The listing builds one solid part. Answer for the finished solid, in the listing's coordinates (mm). A direction names the side the tool comes from. Round coordinates to 2 decimals unless told otherwise and drop trailing zeros. Loops run counter-clockwise (first coordinate to the right, second up) from the corner with the lowest first, then second, coordinate; pieces in that order, holes last. Notation, with made-up numbers: M 7,-19 L 62,-19 A10 cw 62,-14 Z; hole C 53.5,84 d7. An arc over 180 degrees is marked long. Answer as a JSON object with one key per item and string values.
```python
from build123d import *

# Parameters (mm, degrees)
BOSS_EXTRUDE1_DEPTH     = 0.762
SKETCH3_R               = 1.651
SKETCH3_R_2             = 1.1557
BOSS_EXTRUDE2_DEPTH     = 3.175
BOSS_EXTRUDE3_DEPTH     = 0.762
CUT_EXTRUDE1_DEPTH      = 7.703386756
CUT_EXTRUDE1_DEPTH_BACK = 7.703386756
SKETCH5_R               = 1.1557


with BuildPart() as part:
    # Sketch2 → Boss-Extrude1 (new body)
    with BuildSketch(Plane(origin=(0, 0, 0), x_dir=(1, 0, 0), z_dir=(0, 1, 0))):
        with BuildLine():
            ThreePointArc((2.867741935, -1.88005784), (5.08, 0), (2.867741935, 1.88005784))
            ThreePointArc((2.867741935, 1.88005784), (0, 1.647264347), (-2.867741935, 1.88005784))
            ThreePointArc((-2.867741935, 1.88005784), (-5.08, 0), (-2.867741935, -1.88005784))
            ThreePointArc((-2.867741935, -1.88005784), (0, -1.647264347), (2.867741935, -1.88005784))
        make_face()
    extrude(amount=BOSS_EXTRUDE1_DEPTH)

    # Sketch3 → Boss-Extrude2 (add)
    # profile 1 of 2: a face of its own
    with BuildSketch(Plane(origin=(0, 0.762, 0), x_dir=(1, 0, 0), z_dir=(0, 1, 0))):
        with Locations(Location((-3.175, 0, 0), (0, 0, 270))):
            Circle(SKETCH3_R)
        with Locations(Location((-3.175, 0, 0), (0, 0, 270))):
            Circle(SKETCH3_R_2, mode=Mode.SUBTRACT)
    # profile 2 of 2: a face of its own
    with BuildSketch(Plane(origin=(0, 0.762, 0), x_dir=(1, 0, 0), z_dir=(0, 1, 0))):
        with Locations(Location((3.175, 0, 0), (0, 0, 270))):
            Circle(SKETCH3_R)
        with Locations(Location((3.175, 0, 0), (0, 0, 270))):
            Circle(SKETCH3_R_2, mode=Mode.SUBTRACT)
    extrude(amount=BOSS_EXTRUDE2_DEPTH)

    # Sketch4 → Boss-Extrude3 (add)
    with BuildSketch(Plane(origin=(0, 3.937, 0), x_dir=(1, 0, 0), z_dir=(0, 1, 0))):
        with BuildLine():
            ThreePointArc((2.867741935, -1.88005784), (0, -1.647264347), (-2.867741935, -1.88005784))
            ThreePointArc((-2.867741935, -1.88005784), (-5.08, 0), (-2.867741935, 1.88005784))
            ThreePointArc((-2.867741935, 1.88005784), (0, 1.647264347), (2.867741935, 1.88005784))
            ThreePointArc((2.867741935, 1.88005784), (5.08, 0), (2.867741935, -1.88005784))
        make_face()
    extrude(amount=BOSS_EXTRUDE3_DEPTH)

    # Sketch5 → Cut-Extrude1 (cut, two sides: drawn at the far end of the back side and taken through both)
    with BuildSketch(Plane(origin=(0, 0.762, 0), x_dir=(1, 0, 0), z_dir=(0, 1, 0)).offset(-CUT_EXTRUDE1_DEPTH_BACK)):
        with Locations(Location((3.175, 0, 0), (0, 0, 270))):
            Circle(SKETCH5_R)
        with Locations(Location((-3.175, 0, 0), (0, 0, 270))):
            Circle(SKETCH5_R)
    extrude(amount=CUT_EXTRUDE1_DEPTH + CUT_EXTRUDE1_DEPTH_BACK, mode=Mode.SUBTRACT)


solid = part.part
```
Item 1: The part is cut by section A-A (z = 0). Give the vertices of the cut face in (x, y), then the cut area to 3 significant figures.
Values follow:
{"outline": "M -5.08,0 L -4.33,0 L -4.33,4.7 L -5.08,4.7 L -5.08,3.94 L -4.83,3.94 L -4.83,0.76 L -5.08,0.76 Z; M -2.02,0 L 2.02,0 L 2.02,4.7 L -2.02,4.7 Z; M 4.33,0 L 5.08,0 L 5.08,0.76 L 4.83,0.76 L 4.83,3.94 L 5.08,3.94 L 5.08,4.7 L 4.33,4.7 Z; hole M -1.52,0.76 L 1.52,0.76 L 1.52,3.94 L -1.52,3.94 Z", "area": "14.7 mm^2"}
Item 2: The part is cut by section C-C (z = 1.75). Give the vertices of the cut face in (x, y), then the cut area to 3 significant figures.
Values follow:
{"outline": "M -3.93,0 L -1.91,0 L -1.91,0.76 L -3.93,0.76 Z; M -3.93,3.94 L -1.91,3.94 L -1.91,4.7 L -3.93,4.7 Z; M 1.91,0 L 3.93,0 L 3.93,0.76 L 1.91,0.76 Z; M 1.91,3.94 L 3.93,3.94 L 3.93,4.7 L 1.91,4.7 Z", "area": "6.15 mm^2"}
Item 3: The part is cut by section D-D (y = 1.8). Give the vertices of the cut face in (x, z) (3 decimals), then the cut area to 3 significant figures.
Values follow:
{"outline": "C -3.175,0 d3.302; C 3.175,0 d3.302; hole C -3.175,0 d2.311; hole C 3.175,0 d2.311", "area": "8.73 mm^2"}
Item 4: Flat-ended cylindrical pins translate along their axes: P1, Ø1, axis at y = 2.5, z = -1, coming from the -X side; P2, Ø1.5, axis at x = 1, y = 2.5, coming from the -Z side; P3, Ø1.1, axis at x = -2, z = -1, coming from the -Y side; P4, Ø1, axis at y = 3, z = -1, coming from the +X side. Find the tip coordinate at first contact, or state that the pin passes through.
Values follow:
{"P1": "x = -4.75", "P2": "z = -0.83", "P3": "y = 0", "P4": "x = 4.75"}
Item 5: Which of the six approach directions +Z, -Z, +X, -X, +Y, -Y give full straight-line access (tool end or side, diameter ignored) to faces 1 (the face through (0, 0, 0)), 2 (the face through (0, 0.762, 0))?
Values follow:
{"face 1": "+Z, -Z, +X, -X, -Y", "face 2": "none"}
Item 6: The part is cut by section B-B (x = 4). Give the vertices of the cut face in (y, z).
Values follow:
{"outline": "M 0,-1.72 L 0.76,-1.72 L 0.76,-1.43 L 3.94,-1.43 L 3.94,-1.72 L 4.7,-1.72 L 4.7,-0.81 L 0,-0.81 Z; M 0,0.81 L 4.7,0.81 L 4.7,1.72 L 3.94,1.72 L 3.94,1.43 L 0.76,1.43 L 0.76,1.72 L 0,1.72 Z"}
Item 7: Determine the mould class of faces 3 (the face through (0, 4.699, 0)), 4 (the face through (-5.08, 0.38, -0.05)), 5 (the face through (-2.2, 2.32, 0.62)) for opening direction Z: released by +Z, released by -Z, zero draft, split by the parting line, or undercut.
Values follow:
{"face 3": "zero draft", "face 4": "split by the parting line", "face 5": "undercut"}
Item 8: Straight lines are drawn through the part: line 1 (X direction, y = 3.25, z = 0); line 2 (Y direction, x = -1.5, z = 0.5); line 3 (X direction, y = 3.75, z = -0.75). For each, find the intervals that lie inside material, in ascending order.
Values follow:
{"line 1": "-4.83 to -4.33, -2.02 to -1.52, 1.52 to 2.02, 4.33 to 4.83", "line 2": "0 to 0.76, 3.94 to 4.7", "line 3": "-4.65 to -4.05, -2.3 to -1.7, 1.7 to 2.3, 4.05 to 4.65"}
